Input: part model. Units: mm. Frame: model coordinates. A direction names the side the tool comes from. Coordinates: 2 decimals unless noted, no trailing zeros. Order: outer loops, then holes, each group sorted by start corner. A loop starts at its lowest first (then second) coordinate and runs counter-clockwise, first axis right, second up. Notation, with made-up numbers: (48, 66) - (106, 66) arc R22 ccw to (106, 80) - close; hole circle Ø5 at (30.5, -23.75). An arc over 180 degrees is marked (long way). Answer as CSV lines item,"result". Start each with the question number.
Item 1: Draft query along Y for faces 1 (the flat face through (-2, 18, 23.749)), 2 (the flat face through (-13, 0, 26)), 3 (the flat face through (-13, 3, 50.8)), 4 (the cylindrical face through (-2.32, 28.83, 25.36)). Return one class per face: +Y half, -Y half, draft (parallel to the pull), parting line (faces both ways), or undercut.
Item 2: Access query for faces 5 (the flat face through (-4.572, 26, 25)), 6 (the flat face through (0, 18.2, 27.4)), 7 (the cylindrical face through (-2.32, 11.05, 25.36)), 8 (the flat face through (-2, 26, 19.05)). Directions: +Z, -Z, +X, -X, +Y, -Y. A direction counts if a zero-diameter tool reaches every point of the face in a straight line with its end or side. Return the directions, or none.
Item 3: Section C-C (x = -16.51). Output: boundary loops of the cut face in (y, z), and give its area (3 significant figures).
Item 4: Section D-D (x = -2.25). Output: boundary loops of the cut face in (y, z).
Item 5: Material intervals for line 1 along Z through (x, y) = (-16.51, 3.5); line 2 along X through (y, z) = (19, 20); line 3 along Y through (x, z) = (-4.75, 40), sorted ascending.
Item 6: Section A-A (z = 25.4). Output: boundary loops of the cut face in (x, y), and give its area (3 significant figures).
Item 7: First-contact query: pin 1 (5.5 mm diameter, centred on x = -16.51, z = 15.875, fed in from +Y); pin 2 (5 mm diameter, centred on x = -2.5, y = 20, fed in from -Z); pin 3 (1.4 mm diameter, centred on x = -3, y = 27.5, fed in from +Z). Flat tips, straight axial feed; report the tip coordinate or a pass-through.
Item 8: Section B-B (y = 31.5). Output: boundary loops of the cut face in (x, z), and give its area (3 significant figures).
Autodesk Inventor part; units mm, degrees
ref_plane "YZ Plane" through (0, 0, 0) normal (1, 0, 0) x (0, 1, 0)
ref_plane "XZ Plane" through (0, 0, 0) normal (0, 1, 0) x (-1, 0, 0)
ref_plane "XY Plane" through (0, 0, 0) normal (0, 0, 1) x (1, 0, 0)
sketch "Sketch15" plane through (0, 0, 0) normal (0, 1, 0) x (-1, 0, 0)
  line L0 (0, 0) -> (25.4, 0)
  line L1 (25.4, 0) -> (25.4, 50.8)
  line L2 (25.4, 50.8) -> (0, 50.8)
  line L3 (0, 50.8) -> (0, 0)
  dimension "d64" = 25.4
  dimension "d65" = 50.8
extrude "Extrusion12" add sketch "Sketch15" along normal blind 6.35
sketch "Sketch17" plane through (0, 6.35, 0) normal (0, 1, 0) x (1, 0, 0)
  line L0 (-25.4, 0) -> (-25.4, -50.8)
  line L1 (-25.4, -50.8) -> (0, -50.8)
  line L2 (0, -50.8) -> (0, 0)
  line L3 (0, 0) -> (-25.4, 0)
  line L4 (0, -25.4) -> (0, -19.05)
  line L5 (0, -25.4) -> (0, -31.75)
  line L6 (0, -31.75) -> (-4.572, -31.75)
  line L7 (-4.572, -31.75) -> (0, -31.75)
  line L8 (0, -31.75) -> (0, -19.05)
  line L9 (0, -19.05) -> (-4.572, -19.05)
  line L10 (-4.572, -19.05) -> (-4.572, -31.75)
  dimension "d74" = 6.35
  dimension "d75" = 6.35
  dimension "d76" = 4.572
extrude "Extrusion14" add sketch "Sketch17" along normal blind 40.64 contours L2 L6 L10 L9
sketch "Sketch18" plane through (-4.572, 6.35, 19.05) normal (-1, 0, 0) x (0, 0, 1)
  line L0 (12.7, 0) -> (0, 0)
  line L1 (12.7, 0) -> (12.7, 40.64)
  line L2 (0, 40.64) -> (12.7, 40.64)
  line L3 (0, 0) -> (0, 40.64)
  line L4 (0, 20.32) -> (12.7, 20.32) construction
  line L5 (6.35, 20.32) -> (6.35, 24.13) construction
  line L6 (6.35, 24.13) -> (6.35, 34.29) construction
  line L7 (8.001, 24.13) -> (8.001, 34.29)
  line L8 (4.699, 34.29) -> (4.699, 24.13)
  arc A0 (4.699, 24.13) -> (8.001, 24.13) centre (6.35, 24.13) ccw
  arc A1 (8.001, 34.29) -> (4.699, 34.29) centre (6.35, 34.29) ccw
  line L9 (8.001, 16.51) -> (8.001, 6.35)
  line L10 (4.699, 6.35) -> (4.699, 16.51)
  arc A2 (8.001, 16.51) -> (4.699, 16.51) centre (6.35, 16.51) ccw
  arc A3 (4.699, 6.35) -> (8.001, 6.35) centre (6.35, 6.35) ccw
  point P0 (-19.05, -6.35)
  point P1 (6.35, 29.21)
  dimension "d79" = 3.81
  dimension "d80" = 10.16
  dimension "d81" = 3.302
extrude "Extrusion15" cut sketch "Sketch18" against normal up to next contours A0 L8 A1 L7 | L9 A3 L10 A2
sketch "Sketch19" plane through (0, 6.35, 0) normal (0, 1, 0) x (1, 0, 0)
  line L0 (-4.572, -19.05) -> (0, -19.05)
  line L1 (0, -19.05) -> (0, 0)
  line L2 (0, 0) -> (-25.4, 0)
  line L3 (-25.4, 0) -> (-25.4, -50.8)
  line L4 (-25.4, -50.8) -> (0, -50.8)
  line L5 (0, -50.8) -> (0, -31.75)
  line L6 (0, -31.75) -> (-4.572, -31.75)
  line L7 (-4.572, -31.75) -> (-4.572, -19.05)
  line L8 (-25.4, -25.4) -> (0, -25.4) construction
  line L9 (0, -50.8) -> (0, 0)
  line L10 (-12.7, -25.4) -> (-16.51, -25.4)
  line L11 (-16.51, -25.4) -> (-16.51, -15.875) construction
  circle A0 centre (-16.51, -15.875) radius 2.413
  line L12 (-16.51, -25.4) -> (-16.51, -34.925) construction
  circle A1 centre (-16.51, -34.925) radius 2.413
  dimension "d84" = 3.81
  dimension "d85" = 9.525
  dimension "d86" = 4.826
extrude "Extrusion16" cut sketch "Sketch19" against normal up to next contours A0 | A1
equation "\"base_thickness\" = 6.35"
equation "\"motor_adapter_width\" = 19.05"
equation "\"d16\" = 0.5 * motor_adapter_width"
equation "\"motor_adapter_across\" = 21.59"
equation "\"motor_u_adapterthickness\" = 3.81"
properties part number "motor_u_adapter"
Determined:
1,face 1,"undercut"
1,face 2,"-Y half"
1,face 3,"draft"
1,face 4,"undercut"
2,face 5,"+Z, -Z, -X, +Y"
2,face 6,"+Z, -Z, +X, +Y, -Y"
2,face 7,"+X, -X"
2,face 8,"-Z, +X, -X, +Y"
3,outline,"(0, 0) - (6.35, 0) - (6.35, 13.46) - (0, 13.46) - close; (0, 18.29) - (6.35, 18.29) - (6.35, 32.51) - (0, 32.51) - close; (0, 37.34) - (6.35, 37.34) - (6.35, 50.8) - (0, 50.8) - close"
3,area,"261 mm^2"
4,outline,"(0, 0) - (6.35, 0) - (6.35, 19.05) - (46.99, 19.05) - (46.99, 31.75) - (6.35, 31.75) - (6.35, 50.8) - (0, 50.8) - close; hole (12.7, 23.75) - (22.86, 23.75) arc R1.65 ccw to (22.86, 27.05) - (12.7, 27.05) arc R1.65 ccw to start; hole (30.48, 23.75) - (40.64, 23.75) arc R1.65 ccw to (40.64, 27.05) - (30.48, 27.05) arc R1.65 ccw to start"
5,line 1,"z = 0 to 13.46, 18.29 to 32.51, 37.34 to 50.8"
5,line 2,"x = -4.57 to 0"
5,line 3,"y = 0 to 6.35"
6,outline,"(-25.4, 0) - (0, 0) - (0, 11.05) - (-4.57, 11.05) - (-4.57, 6.35) - (-25.4, 6.35) - close; (-4.57, 24.51) - (0, 24.51) - (0, 28.83) - (-4.57, 28.83) - close; (-4.57, 42.29) - (0, 42.29) - (0, 46.99) - (-4.57, 46.99) - close"
6,area,"224 mm^2"
7,pin 1,"stops at y = 6.35"
7,pin 2,"stops at z = 19.05"
7,pin 3,"stops at z = 31.75"
8,outline,"(-4.57, 19.05) - (0, 19.05) - (0, 23.75) - (-4.57, 23.75) - close; (-4.57, 27.05) - (0, 27.05) - (0, 31.75) - (-4.57, 31.75) - close"
8,area,"43.0 mm^2"
